```python
from build123d import *

# Parameters (mm, degrees)
SKETCH_1_W               = 30
SKETCH_1_H               = 30
EXTRUDE_1_DEPTH          = 50
SKETCH_2_W               = 28
SKETCH_2_H               = 28
CUT_EXTRUDE_1_DEPTH      = 1
CUT_EXTRUDE_1_DEPTH_BACK = 101
SKETCH_3_R               = 2.025
CUT_EXTRUDE_2_DEPTH      = 1
SKETCH_4_W               = 18
SKETCH_4_H               = 18
CUT_EXTRUDE_3_DEPTH      = 1
FILLET_1_R               = 2
CUT_EXTRUDE_START        = -2
SKETCH_5_R               = 2.025
CUT_EXTRUDE_5_DEPTH      = 32
SKETCH_6_R               = 2.025
CUT_EXTRUDE_6_DEPTH      = 1
CUT_EXTRUDE_6_DEPTH_BACK = 31
SKETCH_7_R               = 7.5
CUT_EXTRUDE_7_DEPTH      = 1
CUT_EXTRUDE_7_DEPTH_BACK = 31
SKETCH_8_R               = 2.025
CUT_EXTRUDE_8_DEPTH      = 1
CUT_EXTRUDE_8_DEPTH_BACK = 31
SKETCH_9_R               = 2.25
EXTRUDE_2_DEPTH          = 1
SKETCH_10_R              = 2.5
EXTRUDE_3_DEPTH          = 1
SKETCH_11_R              = 2.025
CUT_EXTRUDE_9_DEPTH      = 1
CUT_EXTRUDE_9_DEPTH_BACK = 31
SKETCH_12_R              = 2.5
EXTRUDE_4_DEPTH          = 1
CUT_EXTRUDE_10_REACH     = 32
SKETCH_13_R              = 2.525


with BuildPart() as part:
    # 草图1 → 凸台-拉伸1 (new body, symmetric)
    with BuildSketch(Plane.XY):
        Rectangle(SKETCH_1_W, SKETCH_1_H)
    extrude(amount=EXTRUDE_1_DEPTH, both=True)

    # 草图2 → 切除-拉伸1 (cut, two sides)
    with BuildSketch(Plane.XY.offset(50)) as cut_extrude_1_sk:
        Rectangle(SKETCH_2_W, SKETCH_2_H)
    extrude(amount=CUT_EXTRUDE_1_DEPTH, mode=Mode.SUBTRACT)
    extrude(cut_extrude_1_sk.sketch, amount=-CUT_EXTRUDE_1_DEPTH_BACK, mode=Mode.SUBTRACT)

    # 草图3 → 切除-拉伸2 (cut)
    with BuildSketch(Plane.ZY.offset(15)):
        with Locations((10, 0)):
            Circle(SKETCH_3_R)
        with Locations((35, 0)):
            Circle(SKETCH_3_R)
    extrude(amount=-CUT_EXTRUDE_2_DEPTH, mode=Mode.SUBTRACT)

    # 草图4 → 切除-拉伸3 (cut)
    with BuildSketch(Plane.ZY.offset(-14)):
        with Locations((10, 0)):
            Rectangle(SKETCH_4_W, SKETCH_4_H)
    extrude(amount=-CUT_EXTRUDE_3_DEPTH, mode=Mode.SUBTRACT)

    # 圆角1
    fillet_1_edges = [part.edges().sort_by_distance(p)[0] for p in [
        (14.5, 9, 19),
        (14.5, -9, 19),
        (14.5, -9, 1),
        (14.5, 9, 1),
    ]]
    fillet(fillet_1_edges, radius=FILLET_1_R)

    # 草图5 → 切除-拉伸5 (cut)
    with BuildSketch(Plane(origin=(0, -14, 0), x_dir=(1, 0, 0), z_dir=(0, 1, 0)).offset(CUT_EXTRUDE_START)):
        with Locations((-10, -27.5)):
            Circle(SKETCH_5_R)
        with Locations((-10, -42.5)):
            Circle(SKETCH_5_R)
    cut_extrude_5 = extrude(amount=CUT_EXTRUDE_5_DEPTH, mode=Mode.SUBTRACT)

    # 镜向1: 切除-拉伸5 across plane
    add(cut_extrude_5.mirror(Plane(origin=(0, 0, 0), x_dir=(0, 0, 1), z_dir=(1, 0, 0))), mode=Mode.SUBTRACT)

    # 草图6 → 切除-拉伸6 (cut, two sides)
    with BuildSketch(Plane.ZY.offset(15)) as cut_extrude_6_sk:
        with Locations((35, 0)):
            Circle(SKETCH_6_R)
        with Locations((-20, -7.5)):
            Circle(SKETCH_6_R)
        with Locations((-20, 7.5)):
            Circle(SKETCH_6_R)
    extrude(amount=CUT_EXTRUDE_6_DEPTH, mode=Mode.SUBTRACT)
    extrude(cut_extrude_6_sk.sketch, amount=-CUT_EXTRUDE_6_DEPTH_BACK, mode=Mode.SUBTRACT)

    # 草图7 → 切除-拉伸7 (cut, two sides)
    with BuildSketch(Plane.ZY.offset(15)) as cut_extrude_7_sk:
        with Locations((-36.341476857, 0)):
            Circle(SKETCH_7_R)
    extrude(amount=CUT_EXTRUDE_7_DEPTH, mode=Mode.SUBTRACT)
    extrude(cut_extrude_7_sk.sketch, amount=-CUT_EXTRUDE_7_DEPTH_BACK, mode=Mode.SUBTRACT)

    # 草图8 → 切除-拉伸8 (cut, two sides)
    with BuildSketch(Plane.ZY.offset(15)) as cut_extrude_8_sk:
        with Locations((-10, 7.5)):
            Circle(SKETCH_8_R)
        with Locations((-10, -7.5)):
            Circle(SKETCH_8_R)
    extrude(amount=CUT_EXTRUDE_8_DEPTH, mode=Mode.SUBTRACT)
    extrude(cut_extrude_8_sk.sketch, amount=-CUT_EXTRUDE_8_DEPTH_BACK, mode=Mode.SUBTRACT)

    # 草图9 → 凸台-拉伸2 (add)
    with BuildSketch(Plane(origin=(0, 15, 0), x_dir=(1, 0, 0), z_dir=(0, 1, 0))):
        with Locations((10, -27.5)):
            Circle(SKETCH_9_R)
        with Locations((10, -42.5)):
            Circle(SKETCH_9_R)
    extrude(amount=-EXTRUDE_2_DEPTH)

    # 草图10 → 凸台-拉伸3 (add)
    with BuildSketch(Plane.XZ.offset(15)):
        with Locations((10, 42.5)):
            Circle(SKETCH_10_R)
        with Locations((10, 27.5)):
            Circle(SKETCH_10_R)
    extrude(amount=-EXTRUDE_3_DEPTH)

    # 草图11 → 切除-拉伸9 (cut, two sides)
    with BuildSketch(Plane(origin=(0, 15, 0), x_dir=(1, 0, 0), z_dir=(0, 1, 0))) as cut_extrude_9_sk:
        with Locations((10, -35)):
            Circle(SKETCH_11_R)
    extrude(amount=CUT_EXTRUDE_9_DEPTH, mode=Mode.SUBTRACT)
    extrude(cut_extrude_9_sk.sketch, amount=-CUT_EXTRUDE_9_DEPTH_BACK, mode=Mode.SUBTRACT)

    # 草图12 → 凸台-拉伸4 (add)
    with BuildSketch(Plane(origin=(15, 0, 0), x_dir=(0, 0, -1), z_dir=(1, 0, 0))):
        with Locations((-35, 0)):
            Circle(SKETCH_12_R)
    extrude(amount=-EXTRUDE_4_DEPTH)

    # 草图13 → 切除-拉伸10 (cut, up to next)
    with BuildSketch(Plane(origin=(15, 0, 0), x_dir=(0, 0, -1), z_dir=(1, 0, 0)), mode=Mode.PRIVATE) as cut_extrude_10_sk1:
        with Locations((-35, 2.75)):
            Circle(SKETCH_13_R)
    cut_extrude_10_tool1 = extrude(cut_extrude_10_sk1.sketch, amount=-CUT_EXTRUDE_10_REACH, mode=Mode.PRIVATE) & part.part
    add(cut_extrude_10_tool1.solids().sort_by_distance((15, 2.75, 35))[0], mode=Mode.SUBTRACT)


solid = part.part
```
Could you check a few things on this model? Use its own coordinates, in mm. A direction names the side the tool comes from. Coordinates: 2 decimals unless noted, no trailing zeros. Loops run counter-clockwise (first coordinate to the right, second up) from the corner with the lowest first, then second, coordinate; pieces in that order, holes last.
1) Imagine slicing it at A-A (z = 10). List the corners of the cut face in (x, y) for me (3 decimals), and give its area (4 significant figures).
Reported:
outline: (-15, -15) - (15, -15) - (15, -9) - (14, -9) - (14, -14) - (-14, -14) - (-14, -2.025) - (-15, -2.025) - close; (-15, 2.025) - (-14, 2.025) - (-14, 14) - (14, 14) - (14, 9) - (15, 9) - (15, 15) - (-15, 15) - close
area: 93.95 mm2
2) Thinking about a two-plate mould opening in X: for faces 6 (the face through (-14.507, 5.523, -20.439)), 7 (the face through (-10.26, -14.51, 25.49)), 8 (the face through (-10.26, 14.49, 25.49)), 9 (the face through (-15, 0, 1)), which applies, released by +X, released by -X, zero draft, split by the parting line, or undercut?
Reported:
face 6: zero draft
face 7: undercut
face 8: undercut
face 9: released by -X
3) Imagine slicing it at B-B (x = -10). List the corners of the cut face in (y, z) for me (3 decimals).
Reported:
outline: (-15, -50) - (-14, -50) - (-14, 25.475) - (-15, 25.475) - close; (-15, 29.525) - (-14, 29.525) - (-14, 40.475) - (-15, 40.475) - close; (-15, 44.525) - (-14, 44.525) - (-14, 50) - (-15, 50) - close; (14, -50) - (15, -50) - (15, 25.475) - (14, 25.475) - close; (14, 29.525) - (15, 29.525) - (15, 40.475) - (14, 40.475) - close; (14, 44.525) - (15, 44.525) - (15, 50) - (14, 50) - close
4) Imagine slicing it at D-D (z = -10). List the corners of the cut face in (x, y) for me (3 decimals), and give its area (3 significant figures).
Reported:
outline: (-15, -15) - (15, -15) - (15, -9.525) - (14, -9.525) - (14, -14) - (-14, -14) - (-14, -9.525) - (-15, -9.525) - close; (-15, -5.475) - (-14, -5.475) - (-14, 5.475) - (-15, 5.475) - close; (-15, 9.525) - (-14, 9.525) - (-14, 14) - (14, 14) - (14, 9.525) - (15, 9.525) - (15, 15) - (-15, 15) - close; (14, -5.475) - (15, -5.475) - (15, 5.475) - (14, 5.475) - close
area: 99.8 mm2
5) Which directions (+Z, -Z, +X, -X, +Y, -Y) give clear straight access to the entire face, cutting with the end or side of a thin tool? Please do faces 1 (the face through (-14, 0, 1)), 2 (the face through (-14.51, -0.78, 36.87)), 3 (the face through (0, 15, 1)), 4 (the face through (14.51, 8.4, 1.57)), 5 (the face through (14.49, -8.73, -11.61)).
Reported:
face 1: +Z, -Z
face 2: -X
face 3: +Z, -Z, +X, -X, +Y
face 4: +X
face 5: +X, -X
6) Will these pins go through, and if not, where does the flat tip stop? pin 1 Ø3.5 at (x, z) = (-10, 27.5) entering from +Y; pin 2 Ø3 at (y, z) = (0, 35) entering from -X.
Reported:
pin 1: passes through
pin 2: stops at x = 14
7) Imagine slicing it at C-C (y = -12.5). List the corners of the cut face in (x, z) for me, and give its area (3 significant figures).
Reported:
outline: (-15, -50) - (-14, -50) - (-14, 50) - (-15, 50) - close; (14, -50) - (15, -50) - (15, 50) - (14, 50) - close
area: 200 mm2
8) Please list where these lines run through material, in increasing order: line 1 along Y through (x, z) = (-14.2, -20) (3 decimals); line 2 along X through (y, z) = (12.25, 31).
Reported:
line 1: y = -15 to -9.525, -5.475 to 5.475, 9.525 to 15
line 2: x = -15 to -14, 14 to 15
